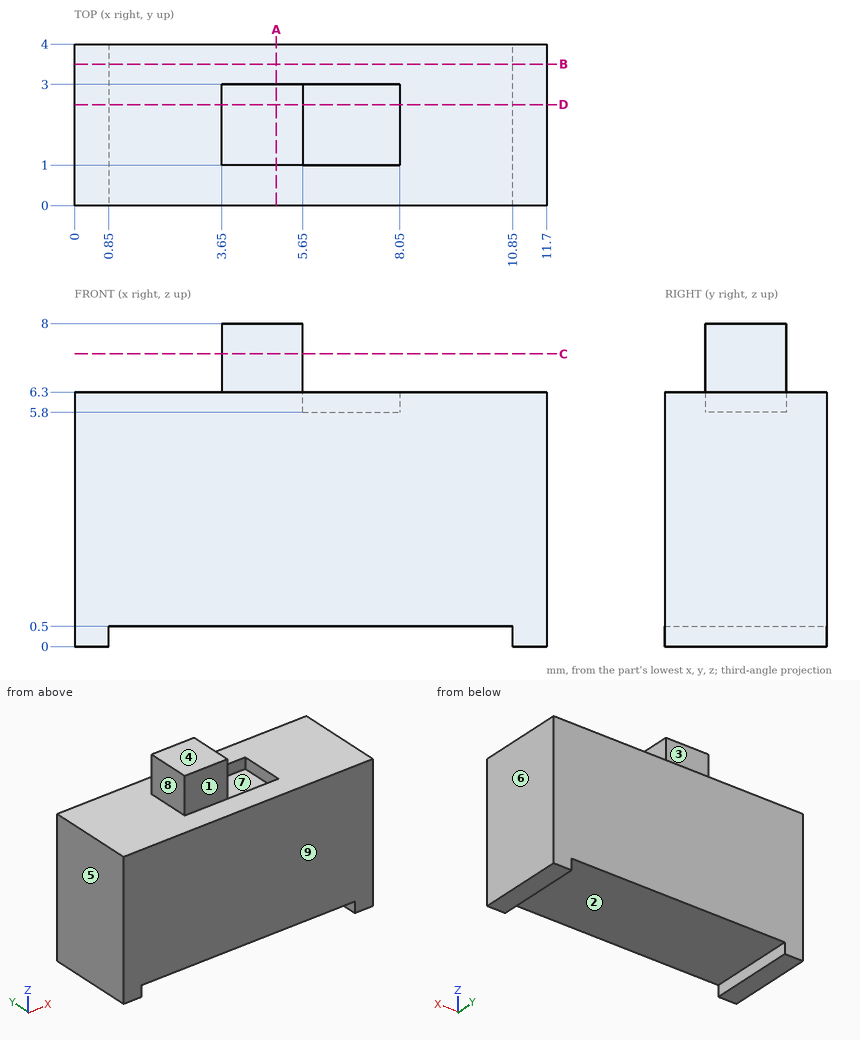
The figure shows three views and two pictorial views of one solid part (mm, origin at its lowest corner). Answer the questions. A direction names the side the tool comes from. Round coordinates to 2 decimals unless told otherwise and drop trailing zeros. Order: outer loops, then holes, each group sorted by start corner. A loop starts at its lowest first (then second) coordinate and runs counter-clockwise, first axis right, second up. Notation, with made-up numbers: M -4,42 L 23,42 A11 cw 23,51 Z; hole C -35.5,8.5 d8. An arc over 180 degrees is marked long. Put each result on its own line as item: value. Start each with the question number.
Q1. Section D-D, the plane y = 2.5 is taken. Write down the section's boundary in (x, z), and give its area (3 significant figures).
Q2. Section A-A, the plane x = 5 is taken. Write down the section's boundary in (y, z).
Q3. Section C-C, the plane z = 7.25 is taken. Write down the section's boundary in (x, y), and give its area (3 significant figures).
Q4. A tool of negligible diameter and unlimited length cuts with its end or side. For the marked faces 1, 2, 3, 4 and 5, from which of +Z, -Z, +X, -X, +Y, -Y can it reach the whole face along a straight path? Write none if from no direction.
Q5. Straight lines are drawn through the part: L1, parallel to Z at x = 9.75, y = 1.55; L2, parallel to Z at x = 11.25, y = 3.15; L3, parallel to X at y = 2.8, z = 7. For each, find the intervals that lie inside material, in ascending order. Write a range as [from, to].
Q6. For a pull along X with two mould halves and no side action, classify the marked faces 6, 7, 8 and 9 as pulls with the +X half, pulls with the -X half, needs draft (parallel to the pull), parting line crosses it, or undercut.
Q7. Section B-B, the plane y = 3.5 is taken. Write down the section's boundary in (x, z).
Q8. Flat-ended cylindrical pins translate along their axes: pin 1 (0.5 mm diameter, centred on y = 2, z = 7, fed in from -X); pin 2 (0.6 mm diameter, centred on y = 2, z = 7.5, fed in from +X); pin 3 (1.4 mm diameter, centred on x = 4.5, z = 7.5, fed in from +Y). Find the tip coordinate at first contact, or state that the pin passes through.
Findings below:
1. outline: M 0,0 L 0.85,0 L 0.85,0.5 L 10.85,0.5 L 10.85,0 L 11.7,0 L 11.7,6.3 L 8.05,6.3 L 8.05,5.8 L 5.65,5.8 L 5.65,8 L 3.65,8 L 3.65,6.3 L 0,6.3 Z
1. area: 70.9 mm^2
2. outline: M 0,0.5 L 4,0.5 L 4,6.3 L 3,6.3 L 3,8 L 1,8 L 1,6.3 L 0,6.3 Z
3. outline: M 3.65,1 L 5.65,1 L 5.65,3 L 3.65,3 Z
3. area: 4.00 mm^2
4. face 1: +Z, +X, -X, -Y
4. face 2: -Z, +Y, -Y
4. face 3: +Z, +X, -X, +Y
4. face 4: +Z, +X, -X, +Y, -Y
4. face 5: +Z, -Z, -X, +Y, -Y
5. L1: z = [0.5, 6.3]
5. L2: z = [0, 6.3]
5. L3: x = [3.65, 5.65]
6. face 6: pulls with the +X half
6. face 7: undercut
6. face 8: pulls with the -X half
6. face 9: needs draft
7. outline: M 0,0 L 0.85,0 L 0.85,0.5 L 10.85,0.5 L 10.85,0 L 11.7,0 L 11.7,6.3 L 0,6.3 Z
8. pin 1: stops at x = 3.65
8. pin 2: stops at x = 5.65
8. pin 3: stops at y = 3
